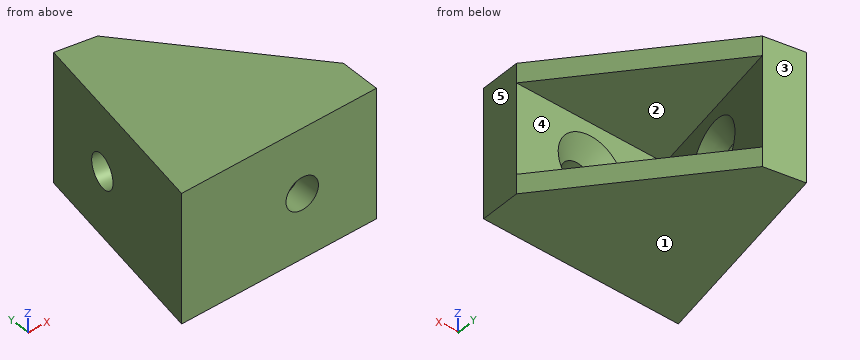
from build123d import *

# Parameters (mm, degrees)
BOSS_EXTRUDE1_DEPTH = 10
BOSS_EXTRUDE2_DEPTH = 3
SKETCH3_R           = 2.5
CUT_EXTRUDE1_DEPTH  = 41.198190433
SKETCH4_R           = 2.5
CUT_EXTRUDE2_DEPTH  = 40.425003339
CHAMFER1_SIZE       = 2.5


with BuildPart() as part:
    # Sketch1 → Boss-Extrude1 (new, symmetric)
    with BuildSketch(Plane.XY):
        Polygon((0, 0), (5.20944533, 29.54423259), (11.118291848, 28.502343524), (7.150521556, 6), (30, 6), (30, 0), align=None)
    extrude(amount=BOSS_EXTRUDE1_DEPTH, both=True)

    # Sketch2 → Boss-Extrude2 (add)
    with BuildSketch(Plane.XY.offset(10)):
        Polygon((11.118291848, 28.502343524), (7.150521556, 6), (30, 6), align=None)
    boss_extrude2 = extrude(amount=-BOSS_EXTRUDE2_DEPTH)

    # Mirror1: Boss-Extrude2 across plane
    add(boss_extrude2.mirror(Plane.XY))

    # Sketch3 → Cut-Extrude1 (cut, through all)
    with BuildSketch(Plane(origin=(5.908846518, -1.041889066, 0), x_dir=(0, 0, -1), z_dir=(0.9848077530122076, -0.173648177666934, 0))):
        with Locations(Location((0, 18.575260778, 0), (0, 0, 90))):
            Circle(SKETCH3_R)
    extrude(amount=-CUT_EXTRUDE1_DEPTH, mode=Mode.SUBTRACT)

    # Sketch4 → Cut-Extrude2 (cut, through all)
    with BuildSketch(Plane(origin=(0, 6, 0), x_dir=(1, 0, 0), z_dir=(0, 1, 0))):
        with Locations(Location((18.575260778, 0, 0), (0, 0, 270))):
            Circle(SKETCH4_R)
    extrude(amount=-CUT_EXTRUDE2_DEPTH, mode=Mode.SUBTRACT)

    # Chamfer1
    chamfer1_edges = [part.edges().sort_by_distance(p)[0] for p in [
        (8.700286258, 14.78915238, 0),
        (18.575260778, 6, -2.5),
    ]]
    chamfer(chamfer1_edges, length=CHAMFER1_SIZE)


solid = part.part
Read the model definition and answer for the solid it produces. Units are mm, in the model's axes. Face numbers are marked on the shaded views. A direction names the side the tool comes from. Coordinates: 2 decimals unless noted, no trailing zeros. Loops run counter-clockwise (first coordinate to the right, second up) from the corner with the lowest first, then second, coordinate; pieces in that order, holes last. Notation, with made-up numbers: (-38.75, 87.25) -> (-5.75, 87.25) arc R18 cw to (-5.75, 101.25) -> close; hole circle Ø6 at (-34, 73). An arc over 180 degrees is marked (long way). Write item = value, one per line. Start each with the question number.
1) Given P1, Ø1.5, axis at y = 24, z = -2, coming from the +X side; P2, Ø11.5, axis at x = 22.5, y = 18.5, coming from the +Z side; P3, Ø8, axis at x = 18.58, z = 0, coming from the +Y side; P4, Ø2, axis at y = 4, z = -5.5, coming from the -X side, each flat-ended and moving along its own axis, determine where each tip first touches the part or whether it passes through.
2) The mould has two halves that part along Y. Classify the marked faces 3, 4 and 5: pulls with the +Y half, pulls with the -Y half, needs draft (parallel to the pull), parting line crosses it, or undercut.
3) Find the intervals of material crossed by L1, parallel to Z at x = 20, y = 14; L2, parallel to Z at x = 6.5, y = 17.75; L3, parallel to Y at x = 18, z = 6.25, in increasing order. Write a range as from..to.
4) The part is cut by section D-D, the plane y = 2.5. Determine the outline of the cut face in (x, z), plus the area to 3 significant figures.
5) The part is cut by section B-B, the plane y = 11.5. Determine the outline of the cut face in (x, z), plus the area to 3 significant figures.
6) The part is cut by section C-C, the plane z = 0. State how many separate pieces and enclosed holes the cut face has, plus the area to 3 significant figures.
7) For the marked faces 1 and 2, determine the directions among +Z, -Z, +X, -X, +Y, -Y from which every point of the face is accessible in a straight line to the end or side of a thin tool.
8) The part is cut by section A-A, the plane z = -6.5. Determine the outline of the cut face in (x, y).
Result:
q1.P1 = 10.46
q1.P2 = 10
q1.P3 = 5
q1.P4 = 0.53
q2.face_3 = pulls with the +Y half
q2.face_4 = undercut
q2.face_5 = needs draft
q3.L1 = -10..-7, 7..10
q3.L2 = -10..-2.5, 2.5..10
q3.L3 = 0..6
q4.outline = (0.44, -10) -> (30, -10) -> (30, 10) -> (0.44, 10) -> close; hole circle Ø5 at (18.58, 0)
q4.area = 572 mm²
q5.outline = (2.03, -10) -> (25.38, -10) -> (25.38, -7) -> (8.12, -7) -> (8.12, 7) -> (25.38, 7) -> (25.38, 10) -> (2.03, 10) -> close
q5.area = 225 mm²
q6.separate_pieces = 3
q6.enclosed_holes = 0
q6.area = 245 mm²
q7.face_1 = -Z, +X, -X, +Y, -Y
q7.face_2 = +X
q8.outline = (0, 0) -> (30, 0) -> (30, 6) -> (7.15, 6) -> (11.12, 28.5) -> (5.21, 29.54) -> close
